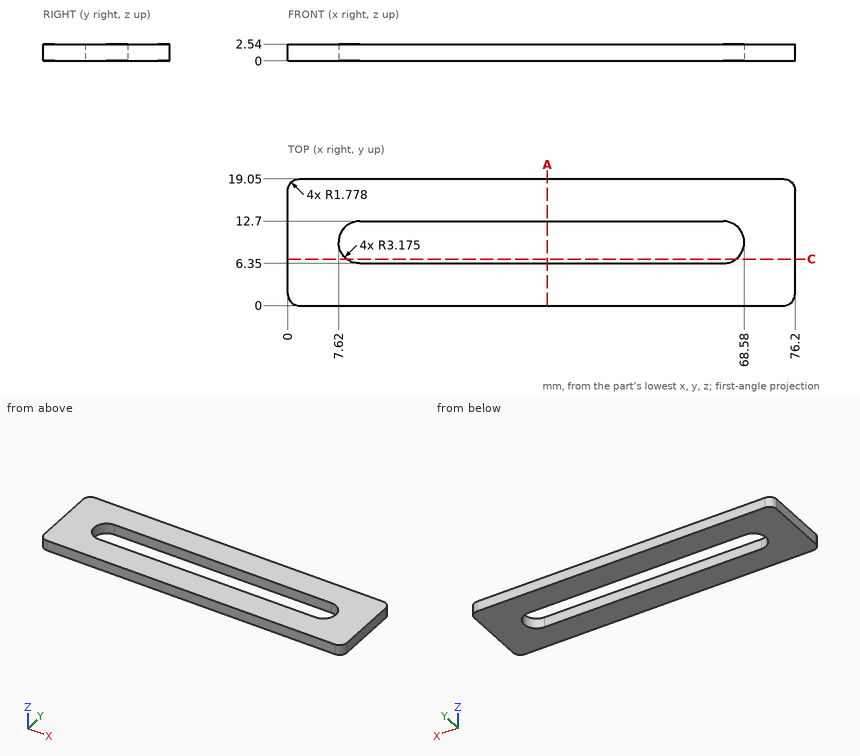
Design review of the part shown in the three views and the two pictorial views. Dimensions are in mm from the part's minimum x, y and z. Coordinates: 2 decimals unless noted, no trailing zeros. Order: outer loops, then holes, each group sorted by start corner. A loop starts at its lowest first (then second) coordinate and runs counter-clockwise, first axis right, second up. Notation, with made-up numbers: (55, 16) -> (105, 16) arc R28 ccw to (105, 34) -> close; hole circle Ø5 at (-8, 59). An arc over 180 degrees is marked (long way). Use one line per item in the form item = value. Start each with the question number.
(1) Add section A-A on x = 39. State the section outline as (y, z) points, plus the area to 3 significant figures.
(2) For probe 1 along Y at (x, z) = (17, 1.95); probe 2 along X at (y, z) = (9.25, 0.65); probe 3 along Y at (x, z) = (10, 2.1), list the stretches that pass through material, from the lowest coordinate up.
(3) Add section C-C on y = 7. State the section outline as (x, z) points.
Answer block:
q1.outline = (0, 0) -> (6.35, 0) -> (6.35, 2.54) -> (0, 2.54) -> close; (12.7, 0) -> (19.05, 0) -> (19.05, 2.54) -> (12.7, 2.54) -> close
q1.area = 32.3 mm²
q2.probe_1 = 0 to 6.35, 12.7 to 19.05
q2.probe_2 = 0 to 7.63, 68.57 to 76.2
q2.probe_3 = 0 to 6.45, 12.6 to 19.05
q3.outline = (0, 0) -> (8.87, 0) -> (8.87, 2.54) -> (0, 2.54) -> close; (67.33, 0) -> (76.2, 0) -> (76.2, 2.54) -> (67.33, 2.54) -> close
